```python
from build123d import *

# Parameters (mm, degrees)
SKETCH1_W           = 42
SKETCH1_H           = 27
SKETCH1_R           = 1.5
BOSS_EXTRUDE1_DEPTH = 2
SKETCH2_R           = 2
SKETCH2_R_2         = 4
SKETCH2_R_3         = 1.5
BOSS_EXTRUDE2_DEPTH = 2
CUT_EXTRUDE1_DEPTH  = 2
FILLET1_R           = 2
FILLET2_R           = 2
FILLET3_R           = 2
FILLET4_R           = 2
FILLET5_R           = 2
BOSS_EXTRUDE3_DEPTH = 2
FILLET6_R           = 2
FILLET7_R           = 2
SKETCH5_R           = 2
CUT_EXTRUDE2_DEPTH  = 2


with BuildPart() as part:
    # Sketch1 → Boss-Extrude1 (new body)
    with BuildSketch(Plane.XY):
        with Locations((21, 13.5)):
            Rectangle(SKETCH1_W, SKETCH1_H)
        with Locations((11, 16)):
            Circle(SKETCH1_R, mode=Mode.SUBTRACT)
        with Locations((11, 23)):
            Circle(SKETCH1_R, mode=Mode.SUBTRACT)
        with Locations((18, 16)):
            Circle(SKETCH1_R, mode=Mode.SUBTRACT)
        with Locations((4, 16)):
            Circle(SKETCH1_R, mode=Mode.SUBTRACT)
        with Locations((11, 9)):
            Circle(SKETCH1_R, mode=Mode.SUBTRACT)
        with Locations((31, 16)):
            Circle(SKETCH1_R, mode=Mode.SUBTRACT)
        with Locations((38, 16)):
            Circle(SKETCH1_R, mode=Mode.SUBTRACT)
        with Locations((31, 23)):
            Circle(SKETCH1_R, mode=Mode.SUBTRACT)
        with Locations((24, 16)):
            Circle(SKETCH1_R, mode=Mode.SUBTRACT)
        with Locations((31, 9)):
            Circle(SKETCH1_R, mode=Mode.SUBTRACT)
    extrude(amount=-BOSS_EXTRUDE1_DEPTH)

    # Sketch2 → Boss-Extrude2 (add)
    with BuildSketch(Plane.XZ):
        with BuildLine():
            Line((0, -32), (0, -36))
            Line((0, -36), (42, -36))
            Line((42, -36), (42, -32))
            Line((42, -32), (50, -32))
            Line((50, -32), (50, -9))
            ThreePointArc((50, -9), (49.414213562, -7.585786438), (48, -7))
            Line((48, -7), (42, -7))
            Line((42, -7), (42, 0))
            Line((42, 0), (0, 0))
            Line((0, 0), (0, -7))
            Line((0, -7), (-6, -7))
            ThreePointArc((-6, -7), (-7.414213562, -7.585786438), (-8, -9))
            Line((-8, -9), (-8, -32))
            Line((-8, -32), (0, -32))
        make_face()
        with Locations((45, -13)):
            Circle(SKETCH2_R, mode=Mode.SUBTRACT)
        with Locations((45, -23)):
            Circle(SKETCH2_R, mode=Mode.SUBTRACT)
        with Locations((-3, -13)):
            Circle(SKETCH2_R, mode=Mode.SUBTRACT)
        with Locations((-3, -23)):
            Circle(SKETCH2_R, mode=Mode.SUBTRACT)
        with Locations((11, -23.5)):
            Circle(SKETCH2_R_2, mode=Mode.SUBTRACT)
        with Locations((31, -23.5)):
            Circle(SKETCH2_R_2, mode=Mode.SUBTRACT)
        with Locations((21, -14.5)):
            Circle(SKETCH2_R_2, mode=Mode.SUBTRACT)
        with Locations((11, -16.5)):
            Circle(SKETCH2_R_3, mode=Mode.SUBTRACT)
        with Locations((11, -30.5)):
            Circle(SKETCH2_R_3, mode=Mode.SUBTRACT)
        with Locations((18, -23.5)):
            Circle(SKETCH2_R_3, mode=Mode.SUBTRACT)
        with Locations((4, -23.5)):
            Circle(SKETCH2_R_3, mode=Mode.SUBTRACT)
        with Locations((31, -30.5)):
            Circle(SKETCH2_R_3, mode=Mode.SUBTRACT)
        with Locations((24, -23.5)):
            Circle(SKETCH2_R_3, mode=Mode.SUBTRACT)
        with Locations((31, -16.5)):
            Circle(SKETCH2_R_3, mode=Mode.SUBTRACT)
        with Locations((38, -23.5)):
            Circle(SKETCH2_R_3, mode=Mode.SUBTRACT)
        with Locations((21, -21.5)):
            Circle(SKETCH2_R_3, mode=Mode.SUBTRACT)
        with Locations((21, -7.5)):
            Circle(SKETCH2_R_3, mode=Mode.SUBTRACT)
        with Locations((28, -14.5)):
            Circle(SKETCH2_R_3, mode=Mode.SUBTRACT)
        with Locations((14, -14.5)):
            Circle(SKETCH2_R_3, mode=Mode.SUBTRACT)
    extrude(amount=-BOSS_EXTRUDE2_DEPTH)

    # Sketch3 → Cut-Extrude1 (cut)
    with BuildSketch(Plane.XZ):
        Polygon((39, -36), (39, -26), (41, -26), (41, -32), (42, -32), (42, -36), align=None)
    cut_extrude1 = extrude(amount=-CUT_EXTRUDE1_DEPTH, mode=Mode.SUBTRACT)

    # Mirror1: Cut-Extrude1 across plane
    add(cut_extrude1.mirror(Plane(origin=(21, 0, 0), x_dir=(0, 0, 1), z_dir=(1, 0, 0))), mode=Mode.SUBTRACT)

    # Fillet1
    fillet1_edges = [part.edges().sort_by_distance(p)[0] for p in [
        (3, 1, -36),
    ]]
    fillet(fillet1_edges, radius=FILLET1_R)

    # Fillet2
    fillet2_edges = [part.edges().sort_by_distance(p)[0] for p in [
        (39, 1, -36),
    ]]
    fillet(fillet2_edges, radius=FILLET2_R)

    # Fillet3
    fillet3_edges = [part.edges().sort_by_distance(p)[0] for p in [
        (21, 0, 0),
    ]]
    fillet(fillet3_edges, radius=FILLET3_R)

    # Fillet4
    fillet4_edges = [part.edges().sort_by_distance(p)[0] for p in [
        (42, 27, -1),
    ]]
    fillet(fillet4_edges, radius=FILLET4_R)

    # Fillet5
    fillet5_edges = [part.edges().sort_by_distance(p)[0] for p in [
        (0, 27, -1),
    ]]
    fillet(fillet5_edges, radius=FILLET5_R)

    # Sketch4 → Boss-Extrude3 (add)
    with BuildSketch(Plane(origin=(0, 0, -32), x_dir=(-1, 0, 0), z_dir=(0, 0, -1))):
        with BuildLine():
            Line((8, 0), (-1, 0))
            Line((-1, 0), (-1, 25))
            ThreePointArc((-1, 25), (-0.414213562, 26.414213562), (1, 27))
            Line((1, 27), (6, 27))
            ThreePointArc((6, 27), (7.414213562, 26.414213562), (8, 25))
            Line((8, 25), (8, 0))
        make_face()
    boss_extrude3 = extrude(amount=-BOSS_EXTRUDE3_DEPTH)

    # Mirror2: Boss-Extrude3 across plane
    add(boss_extrude3.mirror(Plane(origin=(21, 0, 0), x_dir=(0, 0, 1), z_dir=(1, 0, 0))))

    # Fillet6
    fillet6_edges = [part.edges().sort_by_distance(p)[0] for p in [
        (45.5, 0, -32),
    ]]
    fillet(fillet6_edges, radius=FILLET6_R)

    # Fillet7
    fillet7_edges = [part.edges().sort_by_distance(p)[0] for p in [
        (-3.5, 0, -32),
    ]]
    fillet(fillet7_edges, radius=FILLET7_R)

    # Sketch5 → Cut-Extrude2 (cut)
    with BuildSketch(Plane(origin=(0, 0, -32), x_dir=(-1, 0, 0), z_dir=(0, 0, -1))):
        with Locations((3.5, 21)):
            Circle(SKETCH5_R)
        with Locations((3.5, 11)):
            Circle(SKETCH5_R)
    cut_extrude2 = extrude(amount=-CUT_EXTRUDE2_DEPTH, mode=Mode.SUBTRACT)

    # Mirror3: Cut-Extrude2 across plane
    add(cut_extrude2.mirror(Plane(origin=(21, 0, 0), x_dir=(0, 0, 1), z_dir=(1, 0, 0))), mode=Mode.SUBTRACT)


solid = part.part
```
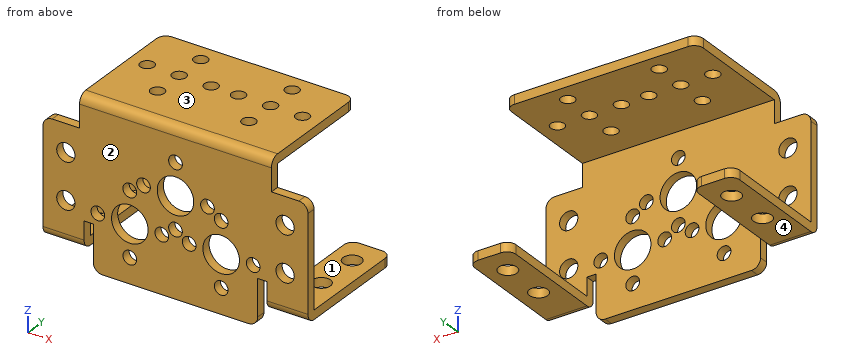
Read the model definition and answer for the solid it produces. Units are mm, in the model's axes. Face numbers are marked on the shaded views. Round coordinates to 2 decimals unless told otherwise and drop trailing zeros. Write each loop counter-clockwise with the first axis right and the second up, starting at its lowest first coordinate (ties: lowest second). Pieces come first, ordered by that corner, then holes. Notation, with made-up numbers: (27, 19) - (64, 19) arc R19 cw to (64, 39) - close; hole circle Ø3 at (52, -8.75). An arc over 180 degrees is marked (long way). One line per item, written item: value.
Q1. Find section C-C (x = 18). Determine the outline of the cut face in (y, z), and give its area (3 significant figures).
The answers:
outline: (0, -36) - (2, -36) - (2, -25) - (0, -25) - close; (0, -22) - (2, -22) - (2, -17.15) - (0, -17.15) - close; (0, -11.85) - (2, -11.85) - (2, -2) - (14.5, -2) - (14.5, 0) - (2, 0) arc R2 ccw to (0, -2) - close; (17.5, -2) - (27, -2) - (27, 0) - (17.5, 0) - close
area: 98.6 mm2
Q2. Find section A-A (x = 11). Count the separate pieces of the cut face and the enclosed holes in it, and give its area (3 significant figures).
The answers:
separate pieces: 7
enclosed holes: 0
area: 75.1 mm2
Q3. For a pull along Z with two mould halves and no side action, classify the marked faces 1, 2, 3 and 4 as pulls with the +Z half, pulls with the -Z half, needs draft (parallel to the pull), parting line crosses it, or undercut.
The answers:
face 1: undercut
face 2: needs draft
face 3: pulls with the +Z half
face 4: pulls with the -Z half
Q4. Each of these flat-tipped pins is pushed along its axis until it touches: P1, Ø2, axis at x = 13.5, y = 16.5, coming from the +Z side; P2, Ø2.5, axis at x = 28, z = -14.5, coming from the -Y side; P3, Ø4, axis at x = 38, z = -23.5, coming from the +Y side; P4, Ø2, axis at x = 31.5, y = 8.5, coming from the -Z side. Where does it stop, or does it pass through?
The answers:
P1: stops at z = 0
P2: passes through
P3: stops at y = 2
P4: stops at z = -2
Q5. Straight lines are drawn through the part: line 1 (Z direction, x = 11, y = 1.65); line 2 (Z direction, x = 25.5, y = 23); line 3 (Z direction, x = -4, y = 25.25). For each, find the intervals that lie inside material, in ascending order. Write a range as from..to.
The answers:
line 1: z = -36..-32, -29..-27.5, -19.5..-18, -15..-0.03
line 2: z = -2..0
line 3: z = -32..-30
Q6. Find section B-B (x = 38). Determine the outline of the cut face in (y, z).
The answers:
outline: (0, -35.73) - (2, -35.73) - (2, -25) - (0, -25) - close; (0, -22) - (2, -22) - (2, -2) - (14.5, -2) - (14.5, 0) - (2, 0) arc R2 ccw to (0, -2) - close; (17.5, -2) - (27, -2) - (27, 0) - (17.5, 0) - close
